Input: part model. Units: mm. Frame: model coordinates. Face numbers are marked on the shaded views. A direction names the side the tool comes from. Round coordinates to 2 decimals unless told otherwise and drop trailing zeros. Write each loop counter-clockwise with the first axis right and the second up, starting at its lowest first coordinate (ties: lowest second). Pieces come first, ordered by that corner, then holes. Notation, with made-up numbers: (84.25, 0.25) -> (128.25, 0.25) arc R29 ccw to (128.25, 37.25) -> close; hole circle Ø6 at (-39, 41.25). An arc over 180 degrees is marked (long way). Write item = value, one per line.
```python
from build123d import *

# Parameters (mm, degrees)
F0_R     = 4.5
F1_DEPTH = 4


with BuildPart() as f1:
    # F0 (on Top) → F1 (new body)
    with BuildSketch(Plane.XY):
        with BuildLine():
            ThreePointArc((-25.367756, 2.593636), (-25.046378, 4.788421), (-24.535476, 6.946973))
            Line((-24.535476, 6.946973), (-26.608073, 6.946973))
            ThreePointArc((-26.608073, 6.946973), (-27.5, 0), (-26.608073, -6.946973))
            Line((-26.608073, -6.946973), (-24.535476, -6.946973))
            ThreePointArc((-24.535476, -6.946973), (-25.046378, -4.788421), (-25.367756, -2.593636))
            ThreePointArc((-25.367756, -2.593636), (-25.5, 0), (-25.367756, 2.593636))
        make_face()
        with BuildLine():
            ThreePointArc((25.367756, 2.593636), (25.466918, 1.298502), (25.5, 0))
            ThreePointArc((25.5, 0), (25.466918, -1.298502), (25.367756, -2.593636))
            ThreePointArc((25.367756, -2.593636), (25.046378, -4.788421), (24.535476, -6.946973))
            Line((24.535476, -6.946973), (26.608073, -6.946973))
            ThreePointArc((26.608073, -6.946973), (27.276107, -3.501998), (27.5, 0))
            ThreePointArc((27.5, 0), (27.276107, 3.501998), (26.608073, 6.946973))
            Line((26.608073, 6.946973), (24.535476, 6.946973))
            ThreePointArc((24.535476, 6.946973), (25.046378, 4.788421), (25.367756, 2.593636))
        make_face()
        with BuildLine():
            ThreePointArc((25.367756, -2.593636), (25.466918, -1.298502), (25.5, 0))
            ThreePointArc((25.5, 0), (25.466918, 1.298502), (25.367756, 2.593636))
            Line((25.367756, 2.593636), (22.867756, 2.593636))
            Line((22.867756, 2.593636), (22.234436, 5.388908))
            ThreePointArc((22.234436, 5.388908), (21.532098, 6.509642), (20.283874, 6.946973))
            Line((20.283874, 6.946973), (0, 6.946973))
            Line((0, 6.946973), (-20.283874, 6.946973))
            ThreePointArc((-20.283874, 6.946973), (-21.532098, 6.509642), (-22.234436, 5.388908))
            Line((-22.234436, 5.388908), (-22.867756, 2.593636))
            Line((-22.867756, 2.593636), (-25.367756, 2.593636))
            ThreePointArc((-25.367756, 2.593636), (-25.5, 0), (-25.367756, -2.593636))
            Line((-25.367756, -2.593636), (-22.867756, -2.593636))
            Line((-22.867756, -2.593636), (-22.234436, -5.388908))
            ThreePointArc((-22.234436, -5.388908), (-21.532098, -6.509642), (-20.283874, -6.946973))
            Line((-20.283874, -6.946973), (0, -6.946973))
            Line((0, -6.946973), (20.283874, -6.946973))
            ThreePointArc((20.283874, -6.946973), (21.532098, -6.509642), (22.234436, -5.388908))
            Line((22.234436, -5.388908), (22.867756, -2.593636))
            Line((22.867756, -2.593636), (25.367756, -2.593636))
        make_face()
        Circle(F0_R, mode=Mode.SUBTRACT)
    extrude(amount=F1_DEPTH)


solid = f1.part
```
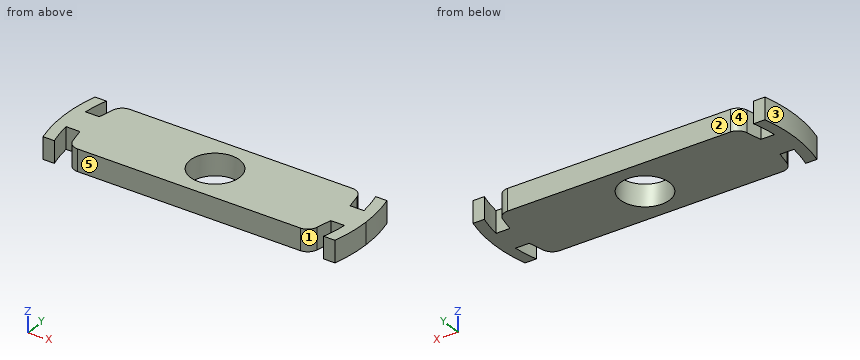
1) Cut plane A-A (z = 1.95). Return the cut outline in (x, y).
Solutions:
outline = (-26.61, -6.95) -> (-24.54, -6.95) arc R25.5 cw to (-25.37, -2.59) -> (-22.87, -2.59) -> (-22.23, -5.39) arc R2 ccw to (-20.28, -6.95) -> (20.28, -6.95) arc R2 ccw to (22.23, -5.39) -> (22.87, -2.59) -> (25.37, -2.59) arc R25.5 cw to (24.54, -6.95) -> (26.61, -6.95) arc R27.5 ccw to (27.5, 0) arc R27.5 ccw to (26.61, 6.95) -> (24.54, 6.95) arc R25.5 cw to (25.37, 2.59) -> (22.87, 2.59) -> (22.23, 5.39) arc R2 ccw to (20.28, 6.95) -> (-20.28, 6.95) arc R2 ccw to (-22.23, 5.39) -> (-22.87, 2.59) -> (-25.37, 2.59) arc R25.5 cw to (-24.54, 6.95) -> (-26.61, 6.95) arc R27.5 ccw to start; hole circle Ø9 at (0, 0)
2) Access query for the marked faces 4 and 5. Directions: +Z, -Z, +X, -X, +Y, -Y. A direction counts if a zero-diameter tool reaches every point of the face in a straight line with its end or side. Return the directions, or none.
Solutions:
face_4 = +Z, -Z, +Y
face_5 = +Z, -Z, +X, -X, -Y
3) Draft query along X for the marked faces 1, 2 and 3. Return one class per face: +X half, -X half, draft (parallel to the pull), parting line (faces both ways), or undercut.
Solutions:
face_1 = undercut
face_2 = draft
face_3 = -X half
4) Cut plane C-C (y = 0.5). Return the cut outline in (x, z).
Solutions:
outline = (-27.5, 0) -> (-4.47, 0) -> (-4.47, 4) -> (-27.5, 4) -> close; (4.47, 0) -> (27.5, 0) -> (27.5, 4) -> (4.47, 4) -> close
5) Cut plane B-B (x = 0). Return the cut outline in (y, z), and give its area (3 significant figures).
Solutions:
outline = (-6.95, 0) -> (-4.5, 0) -> (-4.5, 4) -> (-6.95, 4) -> close; (4.5, 0) -> (6.95, 0) -> (6.95, 4) -> (4.5, 4) -> close
area = 19.6 mm^2
6) First-contact query: P1, Ø0.8, axis at x = 23.5, z = 2, coming from the -Y side; P2, Ø2, axis at y = 4, z = 1.5, coming from the +X side; P3, Ø1.5, axis at y = -1, z = 3.5, coming from the +X side; P4, Ø5.5, axis at x = 0, y = 0, coming from the -Z side. Flat tips, straight axial feed; report the tip coordinate or a pass-through.
Solutions:
P1 = -2.59
P2 = 27.34
P3 = 27.5
P4 = through
7) Cut plane D-D (y = -3.5). Return the cut outline in (x, z), and give its area (3 significant figures).
Solutions:
outline = (-27.28, 0) -> (-25.26, 0) -> (-25.26, 4) -> (-27.28, 4) -> close; (-22.66, 0) -> (-2.83, 0) -> (-2.83, 4) -> (-22.66, 4) -> close; (2.83, 0) -> (22.66, 0) -> (22.66, 4) -> (2.83, 4) -> close; (25.26, 0) -> (27.28, 0) -> (27.28, 4) -> (25.26, 4) -> close
area = 175 mm^2
8) Line query: L1, parallel to Y at x = 0, z = 2.4; L2, parallel to X at y = -3.25, z = 2.25; L3, parallel to X at y = -5.75, z = 3.4. Output: solid intervals per line, ascending. Write a range as from..to.
Solutions:
L1 = -6.95..-4.5, 4.5..6.95
L2 = -27.31..-25.29, -22.72..-3.11, 3.11..22.72, 25.29..27.31
L3 = -26.89..-24.84, -22.12..22.12, 24.84..26.89
